Here's the drawing with two shaded views (mm, measured from the low corner). I have some questions. Round coordinates to 2 decimals unless told otherwise and drop trailing zeros. Write each loop counter-clockwise with the first axis right and the second up, starting at its lowest first coordinate (ties: lowest second). Pieces come first, ordered by that corner, then holes. Notation, with made-up numbers: (-34, -13.75) - (-18, -13.75) arc R32 cw to (-18, 16.25) - close; hole circle Ø1 at (-8, 8.5). An arc over 180 degrees is marked (long way). Return JSON: item names as keys, results as strings. Group by question number.
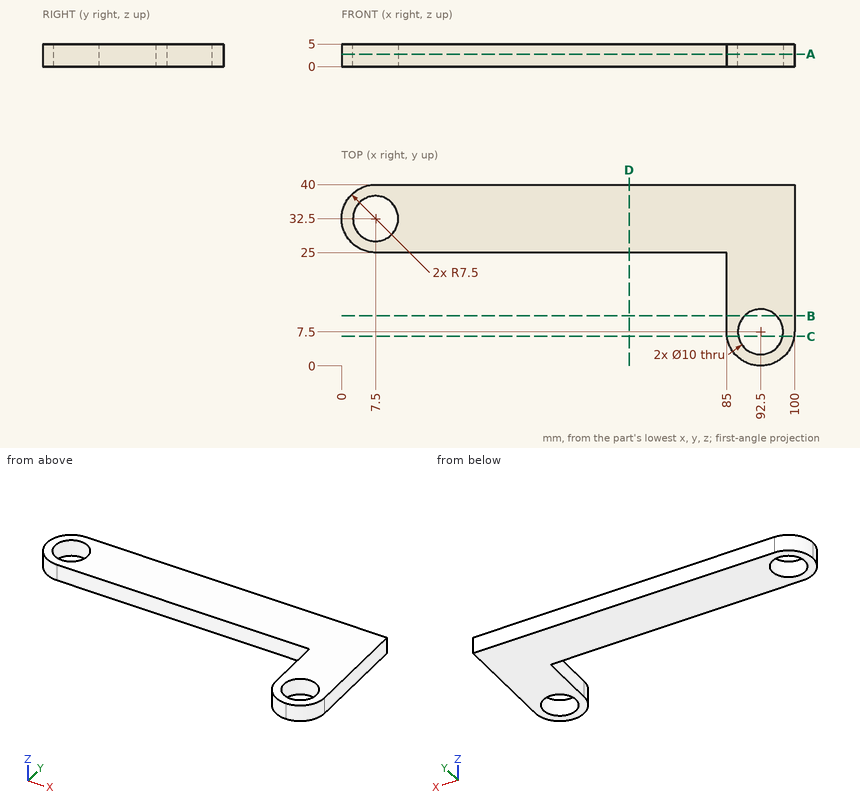
1) I need wall thicknesses on line 1 along Y through (x, z) = (92.5, 1.4); line 2 along Y through (x, z) = (7.5, 3.85); line 3 along X through (y, z) = (16, 2.25). Which ranges of each line are inside material? Lowest first, please.
2) Imagine slicing it at D-D (x = 63.5). Please give me the cut outline in (y, z).
3) Imagine slicing it at A-A (z = 2.75). Please give me the cut outline in (x, y), plus the area to 3 significant figures.
4) Imagine slicing it at B-B (y = 11). Please give me the cut outline in (x, z).
5) Will these pins go through, and if not, where does the flat tip stop? pin 1 Ø11.5 at (x, y) = (92.5, 7.5) entering from +Z; pin 2 Ø1.5 at (y, z) = (12, 3.5) entering from -X.
6) Imagine slicing it at C-C (y = 6.5). Please give me the cut outline in (x, z).
Results found:
{
 "1": {"line 1": "y = 0 to 2.5, 12.5 to 40", "line 2": "y = 25 to 27.5, 37.5 to 40", "line 3": "x = 85 to 100"},
 "2": {"outline": "(25, 0) - (40, 0) - (40, 5) - (25, 5) - close"},
 "3": {"outline": "(7.5, 25) - (85, 25) - (85, 7.5) arc R7.5 ccw to (100, 7.5) - (100, 40) - (7.5, 40) arc R7.5 ccw to start; hole circle Ø10 at (7.5, 32.5); hole circle Ø10 at (92.5, 7.5)", "area": "1,670 mm²"},
 "4": {"outline": "(85, 0) - (88.93, 0) - (88.93, 5) - (85, 5) - close; (96.07, 0) - (100, 0) - (100, 5) - (96.07, 5) - close"},
 "5": {"pin 1": "stops at z = 5", "pin 2": "stops at x = 85"},
 "6": {"outline": "(85.07, 0) - (87.6, 0) - (87.6, 5) - (85.07, 5) - close; (97.4, 0) - (99.93, 0) - (99.93, 5) - (97.4, 5) - close"}
}
